Work out the finished part from the listing and answer in its coordinate system (mm). A direction names the side the tool comes from. Coordinates: 2 decimals unless noted, no trailing zeros. Loops run counter-clockwise (first coordinate to the right, second up) from the corner with the lowest first, then second, coordinate; pieces in that order, holes last. Notation, with made-up numbers: (-32.5, -2) -> (5.5, -2) arc R22 cw to (5.5, 16) -> close; hole circle Ø1 at (32.5, 54.5). An arc over 180 degrees is marked (long way). Answer as CSV lines item,"result".
```python
from build123d import *

# Parameters (mm, degrees)
BOSS_EXTRUDE1_DEPTH = 12.7


with BuildPart() as part:
    # Sketch2 → Boss-Extrude1 (new body)
    with BuildSketch(Plane.XY):
        with BuildLine():
            ThreePointArc((5.773500374, -1.742289015), (0, 6.030661454), (-5.773500374, -1.742289015))
            Line((-5.773500374, -1.742289015), (-8.780460974, -1.742289015))
            ThreePointArc((-8.780460974, -1.742289015), (-8.960066096, -1.667894137), (-9.034460974, -1.488289015))
            Line((-9.034460974, -1.488289015), (-9.034460974, 1.893843998))
            add(Edge.make_bspline(
                [(-7.444124292, 5.87424347), (-8.965547881, 4.023759), (-9.034460974, 1.893843998)],
                knots=[0, 0, 0, 0.913335216, 0.913335216, 0.913335216], degree=2))
            Line((-7.444124292, 5.87424347), (-6.936124292, 5.87424347))
            ThreePointArc((-6.936124292, 5.87424347), (-6.917046287, 5.877961948), (-6.90076124, 5.888573008))
            Line((-6.90076124, 5.888573008), (-6.249346457, 6.52020785))
            ThreePointArc((-6.249346457, 6.52020785), (-6.237627986, 6.575756317), (-6.284709509, 6.607478312))
            Line((-6.284709509, 6.607478312), (-9.286536111, 6.607478312))
            Line((-9.286536111, 6.607478312), (-9.983863182, 6.104225847))
            ThreePointArc((-9.983863182, 6.104225847), (-10.030388572, 5.962190697), (-9.909542054, 5.87424347))
            Line((-9.909542054, 5.87424347), (-8.714124292, 5.87424347))
            add(Edge.make_bspline(
                [(-8.714124292, 5.87424347), (-10.178770924, 3.775549962), (-10.304460974, 1.443821028)],
                knots=[0, 0, 0, 0.841932778, 0.841932778, 0.841932778], degree=2))
            Line((-10.304460974, 1.443821028), (-10.304460974, -2.758289015))
            ThreePointArc((-10.304460974, -2.758289015), (-10.230066096, -2.937894137), (-10.050460974, -3.012289015))
            Line((-10.050460974, -3.012289015), (-5.224460974, -3.012289015))
            ThreePointArc((-5.224460974, -3.012289015), (-4.172972974, -4.353754028), (-2.788146807, -5.347440038))
            ThreePointArc((-2.788146807, -5.347440038), (-2.587836882, -5.362863945), (-2.438222108, -5.228784184))
            Line((-2.438222108, -5.228784184), (-2.117239548, -4.540434863))
            ThreePointArc((-2.117239548, -4.540434863), (-2.106552792, -4.351089815), (-2.22923648, -4.206471467))
            ThreePointArc((-2.22923648, -4.206471467), (0, 4.760661454), (2.22923648, -4.206471467))
            ThreePointArc((2.22923648, -4.206471467), (2.106552792, -4.351089815), (2.117239548, -4.540434863))
            Line((2.117239548, -4.540434863), (2.438222108, -5.228784184))
            ThreePointArc((2.438222108, -5.228784184), (2.587836882, -5.362863945), (2.788146807, -5.347440038))
            ThreePointArc((2.788146807, -5.347440038), (4.172972974, -4.353754028), (5.224460974, -3.012289015))
            Line((5.224460974, -3.012289015), (10.050460974, -3.012289015))
            ThreePointArc((10.050460974, -3.012289015), (10.230066096, -2.937894137), (10.304460974, -2.758289015))
            Line((10.304460974, -2.758289015), (10.304460974, 1.443821028))
            add(Edge.make_bspline(
                [(8.714124292, 5.87424347), (10.178770924, 3.775549962), (10.304460974, 1.443821028)],
                knots=[0, 0, 0, 0.841932778, 0.841932778, 0.841932778], degree=2))
            Line((8.714124292, 5.87424347), (9.909542054, 5.87424347))
            ThreePointArc((9.909542054, 5.87424347), (10.030388572, 5.962190697), (9.983863182, 6.104225847))
            Line((9.983863182, 6.104225847), (9.286536111, 6.607478312))
            Line((9.286536111, 6.607478312), (6.284709509, 6.607478312))
            ThreePointArc((6.284709509, 6.607478312), (6.237627986, 6.575756317), (6.249346457, 6.52020785))
            Line((6.249346457, 6.52020785), (6.90076124, 5.888573008))
            ThreePointArc((6.90076124, 5.888573008), (6.917046287, 5.877961948), (6.936124292, 5.87424347))
            Line((6.936124292, 5.87424347), (7.444124292, 5.87424347))
            add(Edge.make_bspline(
                [(7.444124292, 5.87424347), (8.965547881, 4.023759), (9.034460974, 1.893843998)],
                knots=[0, 0, 0, 0.913335216, 0.913335216, 0.913335216], degree=2))
            Line((9.034460974, 1.893843998), (9.034460974, -1.488289015))
            ThreePointArc((9.034460974, -1.488289015), (8.960066096, -1.667894137), (8.780460974, -1.742289015))
            Line((8.780460974, -1.742289015), (5.773500374, -1.742289015))
        make_face()
    extrude(amount=BOSS_EXTRUDE1_DEPTH)


solid = part.part
```
(1) Consider line 1 along X through (y, z) = (0, 5.25); line 2 along X through (y, z) = (2.5, 8.75); line 3 along Y through (x, z) = (-7.25, 8). Determine where each line is inside the solid, lowest interval first.
Computed values:
line 1,"-10.3 to -9.03, -6.03 to -4.76, 4.76 to 6.03, 9.03 to 10.3"
line 2,"-10.18 to -8.98, -5.49 to -4.05, 4.05 to 5.49, 8.98 to 10.18"
line 3,"-3.01 to -1.74, 5.87 to 6.61"
(2) Flat-ended cylindrical pins translate along their axes: pin 1 Ø1.3 at (x, z) = (-9.5, 8.5) entering from -Y; pin 2 Ø1 at (x, z) = (4.5, 1.5) entering from -Y; pin 3 Ø1.5 at (y, z) = (2.5, 11.5) entering from -X; pin 4 Ø1.5 at (x, y) = (2, -0.5) entering from +Z. Find the tip coordinate at first contact, or state that the pin passes through.
Computed values:
pin 1,"y = -3.01"
pin 2,"y = -4.51"
pin 3,"x = -10.28"
pin 4,"through"
(3) For a pull along Y with two mould halves and no side action, classify faces 1 (the face through (8, 6.607, 6)), 2 (the face through (-0.177, 4.757, 6.261)), 3 (the face through (-2, 5, 12.7)) as pulls with the +Y half, pulls with the -Y half, needs draft (parallel to the pull), parting line crosses it, or undercut.
Computed values:
face 1,"pulls with the +Y half"
face 2,"undercut"
face 3,"needs draft"
(4) A cutting plane is placed at B-B, the plane x = 0. Write down the section's boundary in (y, z).
Computed values:
outline,"(4.76, 0) -> (6.03, 0) -> (6.03, 12.7) -> (4.76, 12.7) -> close"
(5) Which of the six approach directions +Z, -Z, +X, -X, +Y, -Y give full straight-line access (tool end or side, diameter ignored) to faces 4 (the face through (8, -3.012, 6)), 5 (the face through (9, 5.874, 6)), 6 (the face through (-8, -3.012, 6)), 7 (the face through (-7, -1.742, 6))?
Computed values:
face 4,"+Z, -Z, +X, -Y"
face 5,"+Z, -Z, +X"
face 6,"+Z, -Z, -X, -Y"
face 7,"+Z, -Z"
(6) A cutting plane is placed at A-A, the plane y = 0. Write down the section's boundary in (x, z).
Computed values:
outline,"(-10.3, 0) -> (-9.03, 0) -> (-9.03, 12.7) -> (-10.3, 12.7) -> close; (-6.03, 0) -> (-4.76, 0) -> (-4.76, 12.7) -> (-6.03, 12.7) -> close; (4.76, 0) -> (6.03, 0) -> (6.03, 12.7) -> (4.76, 12.7) -> close; (9.03, 0) -> (10.3, 0) -> (10.3, 12.7) -> (9.03, 12.7) -> close"
